CAD build for the part. Positions are in the model's coordinates, mm. Face numbers are marked on the shaded views. Round coordinates to 2 decimals unless told otherwise and drop trailing zeros. Loops run counter-clockwise (first coordinate to the right, second up) from the corner with the lowest first, then second, coordinate; pieces in that order, holes last. Notation, with made-up numbers: (87, 63) -> (101, 63) arc R32 ccw to (101, 101) -> close; hole circle Ø7 at (-30, 14.5). An arc over 180 degrees is marked (long way). Answer as CSV lines item,"result".
```python
from build123d import *

# Parameters (mm, degrees)
BASE_FLANGE3_DEPTH         = 3
SKETCH2_R                  = 3.731705756
CUT_EXTRUDE1_DEPTH         = 10
F_6_0_204_DIAMETER_SLOT2_D = 5.1816
F_6_0_204_DIAMETER_SLOT3_D = 5.1816
F_6_0_204_DIAMETER_SLOT4_D = 5.1816
SKETCH11_R                 = 3.962302528
CUT_EXTRUDE2_DEPTH         = 10


# Sheet-metal steps are written as plain solids
with BuildPart() as part:
    # Sketch1 → Base-Flange3 (new body)
    with BuildSketch(Plane.XY):
        with BuildLine():
            Line((-47.22804279, 44.626403811), (166.055568315, 175.049182627))
            ThreePointArc((166.055568315, 175.049182627), (193.552079509, 168.420316044), (186.923212926, 140.923804851))
            Line((186.923212926, 140.923804851), (-26.360398179, 10.501026034))
            ThreePointArc((-26.360398179, 10.501026034), (-53.856909373, 17.129892617), (-47.22804279, 44.626403811))
        make_face()
    extrude(amount=-BASE_FLANGE3_DEPTH)

    # Sketch2 → Cut-Extrude1 (cut)
    with BuildSketch(Plane.XY):
        with Locations((31.145480049, 80.970292312)):
            Circle(SKETCH2_R)
    extrude(amount=-CUT_EXTRUDE1_DEPTH, mode=Mode.SUBTRACT)

    # #6 (0.204) Diameter Slot2 (through all)
    with Locations(Plane(origin=(0, 0, -3), x_dir=(-1, 0, 0), z_dir=(0, 0, -1))):
        with Locations((-17.407880198, 78.439004647), (-22.671102144, 69.904673863)):
            Hole(F_6_0_204_DIAMETER_SLOT2_D / 2)

    # #6 (0.204) Diameter Slot3 (through all)
    with Locations(Plane(origin=(0, 0, -3), x_dir=(-1, 0, 0), z_dir=(0, 0, -1))):
        with Locations((-56.818082529, 102.219704658), (-61.899947849, 93.651215053)):
            Hole(F_6_0_204_DIAMETER_SLOT3_D / 2)

    # #6 (0.204) Diameter Slot4 (through all)
    with Locations(Plane.XY):
        with Locations((19.820589148, 44.323153185), (14.559362277, 52.969376644), (-19.270561455, 20.579982386), (-24.692774151, 29.137979438)):
            Hole(F_6_0_204_DIAMETER_SLOT4_D / 2)

    # Sketch11 → Cut-Extrude2 (cut)
    with BuildSketch(Plane(origin=(0, 0, -3), x_dir=(-1, 0, 0), z_dir=(0, 0, -1))):
        with Locations((10.804804657, 31.636368095)):
            Circle(SKETCH11_R)
    extrude(amount=-CUT_EXTRUDE2_DEPTH, mode=Mode.SUBTRACT)


solid = part.part
```
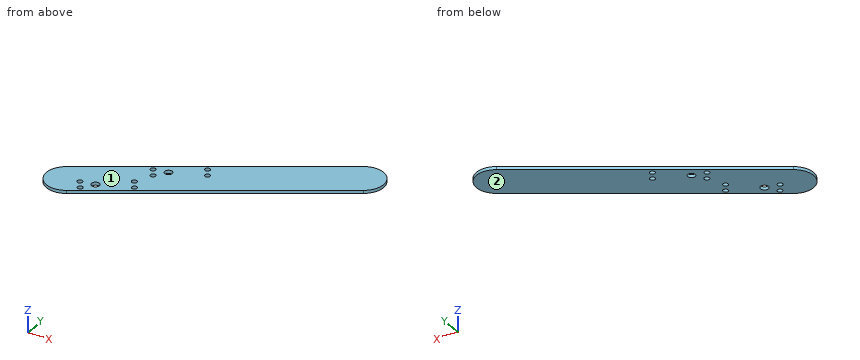
Q1. Slice it at A-A, the plane z = -1.9. Count the separate pieces of the cut face and the enclosed holes in it, and give its area (3 significant figures).
Results:
separate pieces,"1"
enclosed holes,"10"
area,"11,000 mm2"
Q2. Slice it at C-C, the plane x = 76. Give the cut face in (y, z), and give its area (3 significant figures).
Results:
outline,"(73.09, -3) -> (119.98, -3) -> (119.98, 0) -> (73.09, 0) -> close"
area,"141 mm2"
Q3. Two-plate mould, pull along Z, no slides. Class the marked faces 1 and 2: pulls with the +Z half, pulls with the -Z half, needs draft (parallel to the pull), parting line crosses it, or undercut.
Results:
face 1,"pulls with the +Z half"
face 2,"pulls with the -Z half"
Q4. Probe L1, parallel to Y at x = 58, z = -1.3; L2, parallel to X at y = 81.5, z = -1.1; L3, parallel to Y at x = 16, z = -2.5. List the from-to ranges inside material, lowest first. Write a range as [from, to].
Results:
L1,"[62.09, 99.91], [104.53, 108.97]"
L2,"[13.07, 27.45], [34.84, 89.75]"
L3,"[36.4, 50.82], [55.12, 76.26], [80.61, 83.29]"
Q5. Drop flat-ended pins along their axis: pin 1 Ø3 at (x, y) = (-19.27, 20.58) entering from +Z; pin 2 Ø1 at (x, z) = (65.5, -2) entering from +Y. Give the stop position or say it passes through.
Results:
pin 1,"through"
pin 2,"y = 113.87"
Q6. Slice it at B-B, the plane y = 39. Give the cut face in (x, z), and give its area (3 significant figures).
Results:
outline,"(-53.2, -3) -> (20.24, -3) -> (20.24, 0) -> (-53.2, 0) -> close"
area,"220 mm2"
